Here's the drawing with two shaded views (mm, measured from the low corner). I have some questions. A direction names the side the tool comes from. Coordinates: 2 decimals unless noted, no trailing zeros. Write each loop counter-clockwise with the first axis right and the second up, starting at its lowest first coordinate (ties: lowest second). Pieces come first, ordered by that corner, then holes. Notation, with made-up numbers: (-18.5, 71) -> (3.5, 71) arc R28 cw to (3.5, 92) -> close; hole circle Ø10 at (-16.5, 30.5). An arc over 180 degrees is marked (long way). Use one line per item in the form item = value.
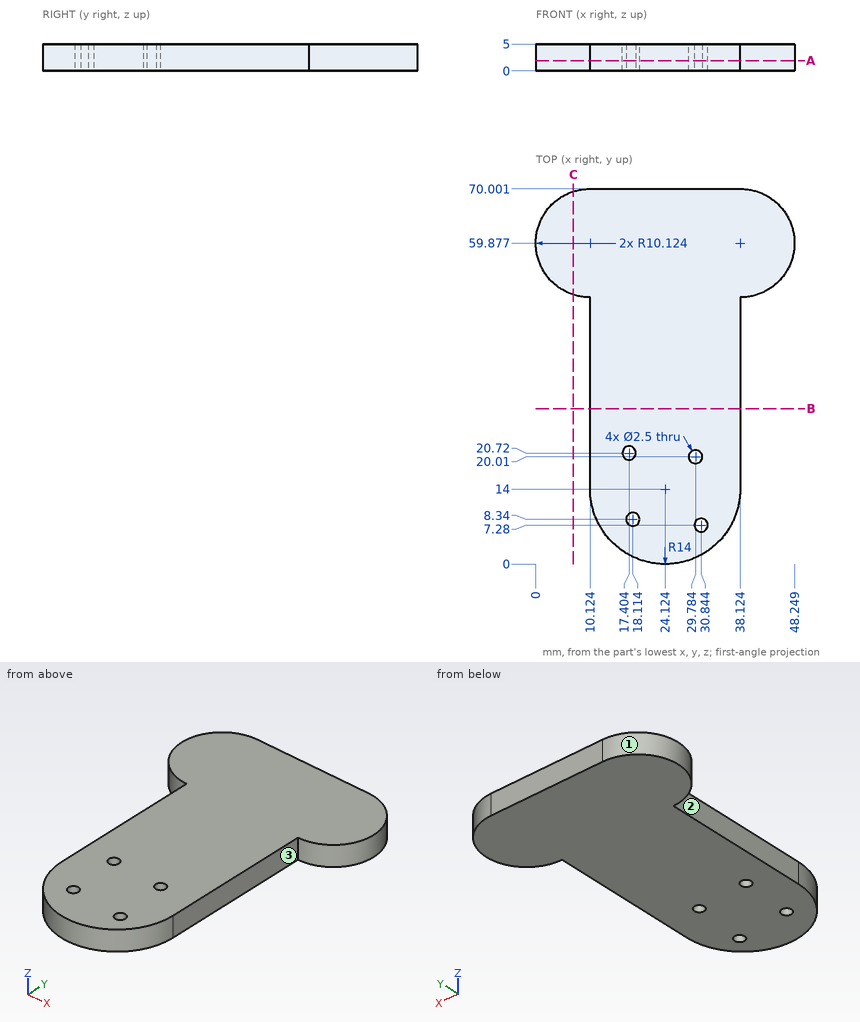
Q1. Suppose I cut it at C-C (x = 7). Write out the boundary of the cut face in (y, z).
Return value:
outline = (50.25, 0) -> (69.51, 0) -> (69.51, 5) -> (50.25, 5) -> close
Q2. Will these pins go through, and if not, where does the flat tip stop? pin 1 (3 mm diameter, centred on y = 7, z = 1, fed in from +X); pin 2 (2 mm diameter, centred on x = 13.5, z = 4, fed in from -Y); pin 3 (1.5 mm diameter, centred on x = 30.84, y = 7.28, fed in from -Z); pin 4 (3 mm diameter, centred on y = 36, z = 4, fed in from +X).
Return value:
pin_1 = 37
pin_2 = 3.83
pin_3 = through
pin_4 = 38.12
Q3. For the marked faces 1, 2 and 3, which set-ups out of +Z, -Z, +X, -X, +Y, -Y let a thin tool reach every point of the face, with its end or its side?
Return value:
face_1 = +Z, -Z, -X
face_2 = +Z, -Z, -X, -Y
face_3 = +Z, -Z, +X, -Y
Q4. If I drill on line 1 (X direction, y = 23.5, z = 1.65) (1 decimal); line 2 (Y direction, x = 19, z = 1.8); line 3 (Y direction, x = 38.5, z = 3.2) (1 decimal), over which ranges is the centre line in solid material (lowest first)? Write a range as from..to.
Return value:
line_1 = 10.1..38.1
line_2 = 0.97..7.46, 9.22..70
line_3 = 49.8..70
Q5. Suppose I cut it at A-A (z = 1.9). Give the number of separate pieces and of enclosed holes in the cut face, then the cut area to 3 significant figures.
Return value:
separate_pieces = 1
enclosed_holes = 4
area = 2,180 mm2
Q6. Suppose I cut it at B-B (y = 29). Write out the boundary of the cut face in (x, z) (1 decimal).
Return value:
outline = (10.1, 0) -> (38.1, 0) -> (38.1, 5) -> (10.1, 5) -> close
